Source: CAD feature listing. Evaluate the final solid. Frame: model axes, mm. A direction names the side the tool comes from. Round coordinates to 2 decimals unless told otherwise and drop trailing zeros. Loops run counter-clockwise (first coordinate to the right, second up) from the corner with the lowest first, then second, coordinate; pieces in that order, holes last. Notation, with made-up numbers: M 35,-18.5 L 81,-18.5 A21 cw 81,15.5 Z; hole C 82,-13 d2. An arc over 180 degrees is marked long. Answer as CSV lines item,"result". Start each with the question number.
Solid Edge part; units mm, degrees
sketch "Sketch1" plane through (0, 0, 0) normal (0, 0, 1) x (1, 0, 0)
  circle A0 centre (0, 0) radius 15.748
  circle A1 centre (0, 0) radius 7.62
extrude "Protrusion1" add sketch "Sketch1" along normal blind 7.366
sketch "Sketch2" plane through (0, 0, 0) normal (0, 0, 1) x (1, 0, 0)
  circle A0 centre (0, -11.684) radius 6.858
extrude "ExtrudedCutout_1" cut sketch "Sketch2" along normal blind 6.858
sketch "Sketch3" plane through (0, 0, 7.366) normal (0, 0, 1) x (1, 0, 0)
  circle A0 centre (0, -11.684) radius 3.683
extrude "ExtrudedCutout_4" cut sketch "Sketch3" against normal blind 4.4355
pattern_circular "Pattern1" count 4 over 360 about axis through (0, 0, 7.366) along (0, 0, 1) of "ExtrudedCutout_4", "ExtrudedCutout_1"
sketch "Sketch4" plane through (0, 0, 7.366) normal (0, 0, 1) x (1, 0, 0)
  circle A0 centre (0, 0) radius 15.748
  circle A1 centre (0, -11.684) radius 3.683
  circle A2 centre (0, 0) radius 7.62
  circle A3 centre (-11.684, 0) radius 3.683
  circle A4 centre (0, 11.684) radius 3.683
  circle A5 centre (11.684, 0) radius 3.683
extrude "ExtrudedProtrusion_7" add sketch "Sketch4" along normal blind 10.795
sketch "Sketch5" plane through (0, 0, 18.161) normal (0, 0, 1) x (1, 0, 0)
  circle A0 centre (0, 0) radius 7.62
extrude "ExtrudedProtrusion_8" add sketch "Sketch5" against normal blind 0.508
sketch "Sketch6" plane through (0, 0, 18.161) normal (0, 0, 1) x (1, 0, 0)
  circle A0 centre (0, 0) radius 18.8759
extrude "ExtrudedCutout_5" cut sketch "Sketch6" against normal blind 6.35
sketch "Sketch7" plane through (0, 0, 11.811) normal (0, 0, 1) x (1, 0, 0)
  circle A0 centre (0, 0) radius 7.62
extrude "ExtrudedProtrusion_9" add sketch "Sketch7" against normal blind 0.508
1) Section A-A, the plane y = 0. Return loops of the section in (x, z).
2) Ray query, line 1 along X through (y, z) = (0, 10.6); line 2 along X through (y, z) = (-1, 11.5). Return the intervals inside material, ascending.
3) Mould query, pull axis Y, two halves, no side actions, for faces 3 (the cylindrical face through (-15.733, -0.692, 7.135)), 4 (the cylindrical face through (10.096, -6.672, 3.381)), 5 (the flat face through (-8, 8, 0)). Classes: pulls with the +Y half, pulls with the -Y half, needs draft (parallel to the pull), parting line crosses it, or undercut.
4) Contact query for flat-ended pins moving along their axis: pin 1 Ø12 at (x, y) = (0, 11.684) entering from -Z; pin 2 Ø2 at (x, y) = (-5, 0) entering from -Z; pin 3 Ø6.5 at (x, y) = (11.684, 0) entering from +Z (1 decimal); pin 4 Ø4 at (x, z) = (6.5, 7) entering from +Y. Output: stop coordinate, or through.
5) Section C-C, the plane y = -9.5. Return loops of the section in (x, z), and give its area (3 significant figures).
6) Access query for faces 1 (the cylindrical face through (0, -8, 9)), 2 (the cylindrical face through (-6.672, -10.096, 3.381)). Directions: +Z, -Z, +X, -X, +Y, -Y. A direction counts if a zero-diameter tool reaches every point of the face in a straight line with its end or side. Return the directions, or none.
7) Section D-D, the plane x = 10. Return loops of the section in (y, z), and give its area (3 significant figures).
Findings below:
1,outline,"M -15.75,6.86 L -15.37,6.86 L -15.37,11.81 L -15.75,11.81 Z; M -8,6.86 L -7.62,6.86 L -7.62,11.3 L 7.62,11.3 L 7.62,6.86 L 8,6.86 L 8,11.81 L -8,11.81 Z; M 15.37,6.86 L 15.75,6.86 L 15.75,11.81 L 15.37,11.81 Z"
2,line 1,"-15.75 to -15.37, -8 to -7.62, 7.62 to 8, 15.37 to 15.75"
2,line 2,"-15.72 to -15.23, -8.14 to 8.14, 15.23 to 15.72"
3,face 3,"parting line crosses it"
3,face 4,"undercut"
3,face 5,"needs draft"
4,pin 1,"z = 6.86"
4,pin 2,"z = 11.3"
4,pin 3,"through"
4,pin 4,"y = 15.09"
5,outline,"M -12.56,0 L -6.5,0 L -6.5,6.86 L -2.97,6.86 L -2.97,11.81 L -12.56,11.81 Z; M 2.97,6.86 L 6.5,6.86 L 6.5,0 L 12.56,0 L 12.56,11.81 L 2.97,11.81 Z"
5,area,"178 mm²"
6,face 1,"+Z, -Z"
6,face 2,"-Z"
7,outline,"M -12.17,0 L -6.65,0 L -6.65,6.86 L -3.28,6.86 L -3.28,11.81 L -12.17,11.81 Z; M 3.28,6.86 L 6.65,6.86 L 6.65,0 L 12.17,0 L 12.17,11.81 L 3.28,11.81 Z"
7,area,"164 mm²"
